from build123d import *

# Parameters (mm, degrees)
BOSS_EXTRU_1_DEPTH      = 6
ENL_V_MAT_EXTRU_1_DEPTH = 6


with BuildPart() as part:
    # Esquisse1 → Boss.-Extru.1 (new body)
    with BuildSketch(Plane(origin=(0, 0, 0), x_dir=(0, 0, -1), z_dir=(1, 0, 0))):
        Polygon((0, 0), (0, 40), (16, 40), (25.775862069, 30.689655172), (29.913793103, 35.034482759), (43.672413793, 21.931034483), (39.534482759, 17.586206897), (58, 0), align=None)
    extrude(amount=BOSS_EXTRU_1_DEPTH)

    # Esquisse2 → Enlèv. mat.-Extru.1 (cut)
    with BuildSketch(Plane(origin=(6, 0, 0), x_dir=(0, 0, -1), z_dir=(1, 0, 0))):
        Polygon((0, 17.5), (0, 12.5), (5, 12.5), (5, 10.7), (10.5, 10.7), (10.5, 12.5), (14.5, 12.5), (14.5, 17.5), (10.5, 17.5), (10.5, 19.3), (5, 19.3), (5, 17.5), align=None)
        Polygon((20.344827586, 35.862068966), (16.724137931, 39.310344828), (13.275862069, 35.689655172), (11.972413793, 36.931034483), (8.179310345, 32.948275862), (9.482758621, 31.706896552), (6.724137931, 28.810344828), (10.344827586, 25.362068966), (13.103448276, 28.25862069), (14.406896552, 27.017241379), (18.2, 31), (16.896551724, 32.24137931), align=None)
    extrude(amount=-ENL_V_MAT_EXTRU_1_DEPTH, mode=Mode.SUBTRACT)


solid = part.part
Can you work these out from the model? Positions are in its coordinate system, mm. A direction names the side the tool comes from. Give positions to 0.01 mm unless a question says otherwise; leave off trailing zeros. Loops run counter-clockwise (first coordinate to the right, second up) from the corner with the lowest first, then second, coordinate; pieces in that order, holes last. Notation, with made-up numbers: (19.5, -29) -> (72.5, -29) arc R12 ccw to (72.5, -25) -> close; hole circle Ø1 at (62.25, 30.25). An arc over 180 degrees is marked (long way). Return JSON: item names as keys, results as strings.
Q1. On a 3-axis mill with a long thin cutter (end or side, diameter ignored), from which of +Z, -Z, +X, -X, +Y, -Y can I reach the whole of each face in a straight line? I mean faces 5 (the face through (2.958, 32.832, -27.816)), 6 (the face through (3, 12.5, -2)), 7 (the face through (2.958, 8.916, -48.638)), 8 (the face through (3.04, 32.34, -8.82)). Say none if no direction works.
Checks:
{"face 5": "+X, -X, +Y", "face 6": "+Z, +X, -X", "face 7": "-Z, +X, -X", "face 8": "+X, -X"}
Q2. For pin 1 Ø2 at (x, y) = (4, 18.5) entering from -Z; pin 2 Ø0.9 at (x, y) = (2, 11.5) entering from -Z; pin 3 Ø1.5 at (x, y) = (4.5, 7.5) entering from -Z, each with a flat end and sliding along its axis, tell me the tip position at first contact or that it passes through.
Checks:
{"pin 1": "stops at z = -41.36", "pin 2": "stops at z = -46.4", "pin 3": "stops at z = -50.91"}
Q3. I want a section at B-B, the plane y = 29.5. List the corners of the cut face in (x, z) for me (3 decimals).
Checks:
{"outline": "(0, -35.725) -> (6, -35.725) -> (6, -16.771) -> (0, -16.771) -> close; (0, -7.381) -> (6, -7.381) -> (6, 0) -> (0, 0) -> close"}
Q4. I want a section at C-C, the plane z = -42. List the corners of the cut face in (x, y) for me (3 decimals), then the cut area to 3 significant figures.
Checks:
{"outline": "(0, 0) -> (6, 0) -> (6, 15.238) -> (0, 15.238) -> close; (0, 20.175) -> (6, 20.175) -> (6, 23.524) -> (0, 23.524) -> close", "area": "112 mm2"}
Q5. I need wall thicknesses on probe 1 along Y at (x, z) = (1.8, -10); probe 2 along Y at (x, z) = (4.5, -3.5); probe 3 along Y at (x, z) = (1.9, -8.5) (3 decimals). Which ranges of each line are inside material? Lowest first, please.
Checks:
{"probe 1": "y = 0 to 10.7, 19.3 to 25.69, 34.86 to 40", "probe 2": "y = 0 to 12.5, 17.5 to 40", "probe 3": "y = 0 to 10.7, 19.3 to 27.119, 30.675 to 32.643, 33.285 to 40"}
Q6. We'd pull the mould along Z, two halves only. Please class faces 1 (the face through (3.042, 28.981, -16.277)), 2 (the face through (3, 12.5, -12)), 3 (the face through (3, 18, -10.5)), 4 (the face through (3, 6, 0)): released by +Z, released by -Z, zero draft, split by the parting line, or undercut.
Checks:
{"face 1": "undercut", "face 2": "zero draft", "face 3": "undercut", "face 4": "released by +Z"}
Q7. I want a section at D-D, the plane y = 7. List the corners of the cut face in (x, z) for me.
Checks:
{"outline": "(0, -50.65) -> (6, -50.65) -> (6, 0) -> (0, 0) -> close"}
